```python
from build123d import *

# Parameters (mm, degrees)
SKETCH_1_W          = 57
SKETCH_1_H          = 57
EXTRUDE_1_DEPTH     = 78
SKETCH_2_R          = 28.5
EXTRUDE_2_DEPTH     = 53
SKETCH_3_R          = 20
EXTRUDE_3_DEPTH     = 2.5
EXTRUDE_4_DEPTH     = 31.5
SKETCH_5_R          = 2
CUT_EXTRUDE_1_DEPTH = 4
SKETCH_6_W          = 57
SKETCH_6_H          = 57
SKETCH_6_R          = 2.6
EXTRUDE_5_DEPTH     = 9.5


with BuildPart() as part:
    # 草图1 → 凸台-拉伸1 (new body)
    with BuildSketch(Plane.XY):
        Rectangle(SKETCH_1_W, SKETCH_1_H)
    extrude(amount=EXTRUDE_1_DEPTH)

    # 草图2 → 凸台-拉伸2 (add)
    with BuildSketch(Plane.XY.offset(78)):
        Circle(SKETCH_2_R)
    extrude(amount=EXTRUDE_2_DEPTH)

    # 草图3 → 凸台-拉伸3 (add)
    with BuildSketch(Plane.XY.offset(131)):
        Circle(SKETCH_3_R)
    extrude(amount=EXTRUDE_3_DEPTH)

    # 草图4 → 凸台-拉伸4 (add)
    with BuildSketch(Plane.XY.offset(133.5)):
        with BuildLine():
            Line((0, 9), (2.5, 9))
            Line((2.5, 9), (2.5, 6.538348415))
            ThreePointArc((2.5, 6.538348415), (0.021437338, -6.999967174), (-2.54, 6.522913459))
            Line((-2.54, 6.522913459), (-2.54, 9))
            Line((-2.54, 9), (0, 9))
        make_face()
    extrude(amount=EXTRUDE_4_DEPTH)

    # 草图5 → 切除-拉伸1 (cut)
    with BuildSketch(Plane.XY.offset(131)):
        with Locations((0, -17.5)):
            Circle(SKETCH_5_R)
        with Locations((-17.5, 0)):
            Circle(SKETCH_5_R)
        with Locations((0, 17.5)):
            Circle(SKETCH_5_R)
        with Locations((17.5, 0)):
            Circle(SKETCH_5_R)
    extrude(amount=-CUT_EXTRUDE_1_DEPTH, mode=Mode.SUBTRACT)

    # 草图6 → 凸台-拉伸5 (add)
    with BuildSketch(Plane.XY.offset(131)):
        Rectangle(SKETCH_6_W, SKETCH_6_H)
        with Locations((-23.57, 23.57)):
            Circle(SKETCH_6_R, mode=Mode.SUBTRACT)
        with Locations((23.57, 23.57)):
            Circle(SKETCH_6_R, mode=Mode.SUBTRACT)
        with Locations((23.57, -23.57)):
            Circle(SKETCH_6_R, mode=Mode.SUBTRACT)
        with Locations((-23.57, -23.57)):
            Circle(SKETCH_6_R, mode=Mode.SUBTRACT)
    extrude(amount=-EXTRUDE_5_DEPTH)


solid = part.part
```
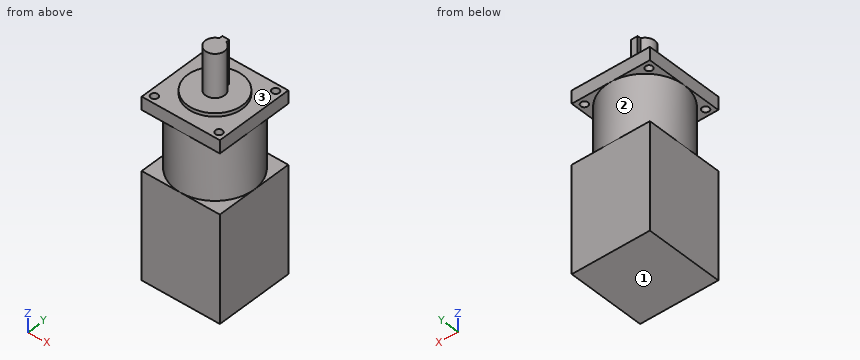
Work out the finished part from the listing and answer in its coordinate system (mm). Face numbers are marked on the shaded views. A direction names the side the tool comes from. Round coordinates to 2 decimals unless told otherwise and drop trailing zeros. Loops run counter-clockwise (first coordinate to the right, second up) from the corner with the lowest first, then second, coordinate; pieces in that order, holes last.
(1) The part is cut by section C-C, the plane z = 98. Give the vertices of the cut face in (x, y), and give its area (3 significant figures).
Computed values:
outline: circle Ø57 at (0, 0)
area: 2,550 mm2
(2) The part is cut by section A-A, the plane y = -23.57. Give the vertices of the cut face in (x, z).
Computed values:
outline: (-28.5, 0) - (28.5, 0) - (28.5, 78) - (16.02, 78) - (16.02, 121.5) - (20.97, 121.5) - (20.97, 131) - (-20.97, 131) - (-20.97, 121.5) - (-16.02, 121.5) - (-16.02, 78) - (-28.5, 78) - close; (-28.5, 121.5) - (-26.17, 121.5) - (-26.17, 131) - (-28.5, 131) - close; (26.17, 121.5) - (28.5, 121.5) - (28.5, 131) - (26.17, 131) - close
(3) Find the intervals of material crossed by L1, parallel to Y at x = 23.57, z = 127; L2, parallel to Z at x = 12.5, y = 26.5; L3, parallel to X at y = 23, z = 127, in increasing order.
Computed values:
L1: y = -28.5 to -26.17, -20.97 to 20.97, 26.17 to 28.5
L2: z = 0 to 78, 121.5 to 131
L3: x = -28.5 to -26.11, -21.03 to 21.03, 26.11 to 28.5
(4) Each of these flat-tipped pins is pushed along its axis until it touches: P1, Ø3, axis at y = -21.5, z = 100.5, coming from the +X side; P2, Ø1.5, axis at y = 17.5, z = 87.5, coming from the +X side; P3, Ø12, axis at y = 13.5, z = 144, coming from the -X side. Where does it stop, or does it pass through?
Computed values:
P1: stops at x = 20.3
P2: stops at x = 23.06
P3: stops at x = -2.54
(5) For the marked faces 1, 2 and 3, determine the directions among +Z, -Z, +X, -X, +Y, -Y from which every point of the face is accessible in a straight line to the end or side of a thin tool.
Computed values:
face 1: -Z, +X, -X, +Y, -Y
face 2: none
face 3: +Z
(6) The part is cut by section D-D, the plane y = 12. Give the vertices of the cut face in (x, z).
Computed values:
outline: (-28.5, 0) - (28.5, 0) - (28.5, 78) - (25.85, 78) - (25.85, 121.5) - (28.5, 121.5) - (28.5, 131) - (16, 131) - (16, 133.5) - (-16, 133.5) - (-16, 131) - (-28.5, 131) - (-28.5, 121.5) - (-25.85, 121.5) - (-25.85, 78) - (-28.5, 78) - close
